```python
from build123d import *
from OCP.BRepFilletAPI import BRepFilletAPI_MakeChamfer

# Parameters (mm, degrees)
BOSS_EXTRUDE1_DEPTH = 0.5
CHAMFER1_SIZE       = 1.27
CHAMFER1_SIZE2      = 0.25
CHAMFER2_SIZE       = 0.25
CHAMFER2_SIZE2      = 1.27


with BuildPart() as part:
    # Sketch1 → Boss-Extrude1 (new, symmetric)
    with BuildSketch(Plane(origin=(0, 0, 0), x_dir=(0, 0, -1), z_dir=(1, 0, 0))):
        with BuildLine():
            Line((0.5, -2), (0.5, -7.62))
            Line((0.5, -7.62), (-0.5, -7.62))
            Line((-0.5, -7.62), (-0.5, -2))
            ThreePointArc((-0.5, -2), (-0.939339828, -0.939339828), (-2, -0.5))
            Line((-2, -0.5), (-8.64, -0.5))
            Line((-8.64, -0.5), (-8.64, 0.5))
            Line((-8.64, 0.5), (-2, 0.5))
            ThreePointArc((-2, 0.5), (-0.232233047, -0.232233047), (0.5, -2))
        make_face()
    extrude(amount=BOSS_EXTRUDE1_DEPTH, both=True)

    # Chamfer1: one chamfer whose edges measure the first distance from different faces: ONE call of the kernel's chamfer builder (chamfer() names one face for all edges)
    chamfer1_edges_1 = [part.edges().sort_by_distance(p)[0] for p in [
        (-0.5, 0, 8.64),
    ]]
    chamfer1_side_1 = [part.faces().sort_by_distance(p)[0] for p in [
        (-0.5, -4.81, -0.37774044),
    ]]
    chamfer1_edges_2 = [part.edges().sort_by_distance(p)[0] for p in [
        (0.5, 0, 8.64),
    ]]
    chamfer1_side_2 = [part.faces().sort_by_distance(p)[0] for p in [
        (0.5, -4.81, -0.37774044),
    ]]
    chamfer1_edges_3 = [part.edges().sort_by_distance(p)[0] for p in [
        (0, -0.5, 8.64),
    ]]
    chamfer1_side_3 = [part.faces().sort_by_distance(p)[0] for p in [
        (0, -0.5, 5.32),
    ]]
    chamfer1_edges_4 = [part.edges().sort_by_distance(p)[0] for p in [
        (0, 0.5, 8.64),
    ]]
    chamfer1_side_4 = [part.faces().sort_by_distance(p)[0] for p in [
        (0, 0.5, 5.32),
    ]]
    chamfer1 = BRepFilletAPI_MakeChamfer(part.part.solid().wrapped)
    for e in chamfer1_edges_1:
        chamfer1.Add(CHAMFER1_SIZE, CHAMFER1_SIZE2, e.wrapped, chamfer1_side_1[0].wrapped)  # the first distance lies on this face
    for e in chamfer1_edges_2:
        chamfer1.Add(CHAMFER1_SIZE, CHAMFER1_SIZE2, e.wrapped, chamfer1_side_2[0].wrapped)  # the first distance lies on this face
    for e in chamfer1_edges_3:
        chamfer1.Add(CHAMFER1_SIZE, CHAMFER1_SIZE2, e.wrapped, chamfer1_side_3[0].wrapped)  # the first distance lies on this face
    for e in chamfer1_edges_4:
        chamfer1.Add(CHAMFER1_SIZE, CHAMFER1_SIZE2, e.wrapped, chamfer1_side_4[0].wrapped)  # the first distance lies on this face
    add(Compound.cast(chamfer1.Shape()), mode=Mode.REPLACE)

    # Chamfer2
    chamfer2_edges = [part.edges().sort_by_distance(p)[0] for p in [
        (0, -7.62, -0.5),
        (0, -7.62, 0.5),
        (0.5, -7.62, 0),
        (-0.5, -7.62, 0),
    ]]
    chamfer2_side = [part.faces().sort_by_distance(p)[0] for p in [
        (0, -7.62, 0),
    ]]
    chamfer(chamfer2_edges, length=CHAMFER2_SIZE, length2=CHAMFER2_SIZE2, reference=chamfer2_side[0])


solid = part.part
```
Read the model definition and answer for the solid it produces. Units are mm, in the model's axes. A direction names the side the tool comes from. Round coordinates to 2 decimals unless told otherwise and drop trailing zeros. Write each loop counter-clockwise with the first axis right and the second up, starting at its lowest first coordinate (ties: lowest second). Pieces come first, ordered by that corner, then holes. Notation, with made-up numbers: (27.5, 70) - (57.5, 70) arc R16 ccw to (57.5, 90) - close; hole circle Ø9 at (5, 73). An arc over 180 degrees is marked (long way). One line per item, written item: value.
Q1. Find section C-C (z = 2.75). Determine the outline of the cut face in (x, y).
The answers:
outline: (-0.5, -0.5) - (0.5, -0.5) - (0.5, 0.5) - (-0.5, 0.5) - close
Q2. This flat-tipped pin is pushed along its axis until it touches: P1, Ø1.5, axis at y = -4.5, z = 2, coming from the +X side. Where does it stop, or does it pass through?
The answers:
P1: passes through
Q3. Find section B-B (y = 0). Determine the outline of the cut face in (x, z), and give its area (3 significant figures).
The answers:
outline: (-0.5, 0.5) - (0.5, 0.5) - (0.5, 7.37) - (0.25, 8.64) - (-0.25, 8.64) - (-0.5, 7.37) - close
area: 7.82 mm2
Q4. Straight lines are drawn through the part: line 1 (Z direction, x = 0.3, y = -6.25); line 2 (Y direction, x = 0.1, z = 0). For each, find the intervals that lie inside material, in ascending order. Write a range as from..to.
The answers:
line 1: z = -0.5..0.5
line 2: y = -7.62..-0.5
Q5. Which of the six approach directions +Z, -Z, +X, -X, +Y, -Y give full straight-line access (tool end or side, diameter ignored) to faces 1 (the flat face through (-0.4, -0.01, 7.87)), 2 (the flat face through (0, -0.5, 5))?
The answers:
face 1: +Z, -X, +Y, -Y
face 2: +Z, +X, -X, -Y
Q6. Find section A-A (x = 0.05). Determine the outline of the cut face in (y, z).
The answers:
outline: (-7.62, -0.25) - (-6.35, -0.5) - (-2, -0.5) arc R2.5 ccw to (0.5, 2) - (0.5, 7.37) - (0.25, 8.64) - (-0.25, 8.64) - (-0.5, 7.37) - (-0.5, 2) arc R1.5 cw to (-2, 0.5) - (-6.35, 0.5) - (-7.62, 0.25) - close
